Autodesk Inventor part; units mm, degrees
ref_plane "Work Plane1" through (15.7004, 0, 0) normal (0, -1, 0) x (1, 0, 0)
ref_plane "YZ Plane" through (0, 0, 0) normal (1, 0, 0) x (0, 1, 0)
ref_plane "XZ Plane" through (0, 0, 0) normal (0, 1, 0) x (-1, 0, 0)
sketch "Sketch1" plane through (0, 0, 0) normal (0, 0, 1) x (1, 0, 0)
  arc A0 (-20.5392, 17.1146) -> (-21.125, 15.7004) centre (-19.125, 15.7004) ccw
  line L0 (-21.125, -15.7004) -> (-21.125, 15.7004)
  arc A1 (-21.125, -15.7004) -> (-20.5392, -17.1146) centre (-19.125, -15.7004) ccw
  line L1 (-20.5392, -17.1146) -> (-17.1146, -20.5392)
  arc A2 (-17.1146, -20.5392) -> (-15.7004, -21.125) centre (-15.7004, -19.125) ccw
  line L2 (15.7004, -21.125) -> (-15.7004, -21.125)
  arc A3 (15.7004, -21.125) -> (17.1146, -20.5392) centre (15.7004, -19.125) ccw
  line L3 (20.5392, -17.1146) -> (17.1146, -20.5392)
  arc A4 (20.5392, -17.1146) -> (21.125, -15.7004) centre (19.125, -15.7004) ccw
  line L4 (21.125, 15.7004) -> (21.125, -15.7004)
  arc A5 (21.125, 15.7004) -> (20.5392, 17.1146) centre (19.125, 15.7004) ccw
  line L5 (20.5392, 17.1146) -> (17.1146, 20.5392)
  arc A6 (17.1146, 20.5392) -> (15.7004, 21.125) centre (15.7004, 19.125) ccw
  line L6 (-15.7004, 21.125) -> (15.7004, 21.125)
  arc A7 (-15.7004, 21.125) -> (-17.1146, 20.5392) centre (-15.7004, 19.125) ccw
  line L7 (-20.5392, 17.1146) -> (-17.1146, 20.5392)
  circle A8 centre (0, 0) radius 16
  circle A9 centre (-15.875, -15.875) radius 1.625
  circle A10 centre (15.875, 15.875) radius 1.625
  circle A11 centre (-15.875, 15.875) radius 1.625
  circle A12 centre (15.875, -15.875) radius 1.625
  circle A13 centre (0, 0) radius 11
  point P0 (0, 0)
extrude "Extrusion1" add sketch "Sketch1" along normal blind 5 contours L7 A7 L6 A6 L5 A5 L4 A4 L3 A3 L2 A2 L1 A1 L0 A0 | A8
sketch "Sketch2" plane through (-21.125, -15.7004, 0) normal (-1, 0, 0) x (0, 0, 1)
  line L0 (0, -5.4246) -> (5, -5.4246)
  line L1 (5, -5.4246) -> (-28, -5.4246)
  line L2 (-28, -5.4246) -> (-28, 36.8254)
  line L3 (-28, 36.8254) -> (5, 36.8254)
  line L4 (5, 36.8254) -> (5, -5.4246)
  point P0 (0, 15.7004)
  dimension "d6" = 33
extrude "Extrusion2" add sketch "Sketch2" along normal blind 5
sketch "Sketch3" plane through (0, 0, 5) normal (0, 0, 1) x (1, 0, 0)
  line L0 (-21.125, -15.7004) -> (-21.125, -21.125)
  arc A0 (-21.125, -15.7004) -> (-20.5392, -17.1146) centre (-19.125, -15.7004) ccw
  arc A1 (-17.1146, -20.5392) -> (-15.7004, -21.125) centre (-15.7004, -19.125) ccw
  line L1 (-20.5392, -17.1146) -> (-17.1146, -20.5392)
  line L2 (-21.125, -21.125) -> (-15.7004, -21.125)
  line L3 (-21.125, 21.125) -> (-21.125, 15.7004)
  arc A2 (-15.7004, 21.125) -> (-17.1146, 20.5392) centre (-15.7004, 19.125) ccw
  line L4 (-21.125, 21.125) -> (-15.7004, 21.125)
  line L5 (-17.1146, 20.5392) -> (-20.5392, 17.1146)
  arc A3 (-20.5392, 17.1146) -> (-21.125, 15.7004) centre (-19.125, 15.7004) ccw
  point P0 (0, 0)
extrude "Extrusion3" add sketch "Sketch3" against normal blind 5
sketch "Sketch4" plane through (-26.125, -15.7004, 0) normal (-1, 0, 0) x (0, 0, 1)
  line L0 (0, -5.4246) -> (-28, -5.4246)
  line L1 (5, 36.8254) -> (-28, 36.8254)
  line L2 (-28, -5.4246) -> (-23, -5.4246)
  line L3 (-23, -5.4246) -> (-23, 36.8254)
  line L4 (-23, 36.8254) -> (-28, 36.8254)
  line L5 (-28, 36.8254) -> (-28, -5.4246)
  point P0 (0, 15.7004)
  dimension "d7" = 5
extrude "Extrusion4" add sketch "Sketch4" along normal blind 15
sketch "Sketch5" plane through (-26.125, -21.125, -23) normal (0, 0, 1) x (1, 0, 0)
  circle A0 centre (-5, 32.25) radius 2.25
  circle A1 centre (-5, 10) radius 2.25
  line L0 (0, 42.25) -> (-15, 42.25)
  line L1 (-15, 0) -> (-15, 42.25)
  line L2 (0, 0) -> (-15, 0)
  point P0 (26.125, 21.125)
  dimension "d10" = 10
  dimension "d11" = 10
  dimension "d12" = 10
  dimension "d13" = 10
  dimension "d14" = 4.5
  dimension "d15" = 4.5
extrude "Extrusion5" cut sketch "Sketch5" along normal through all both and the other way through all
ref_plane "Work Plane1" through (15.7004, 0, 0) normal (0, -1, 0) x (1, 0, 0)
sketch "Sketch6" plane through (15.7004, 0, 0) normal (0, -1, 0) x (1, 0, 0)
  line L0 (-41.8254, -23) -> (-56.8254, -23)
  line L1 (0, 5) -> (-41.8254, 5)
  line L2 (-56.8254, -23) -> (-41.8254, 5)
  line L3 (-41.8254, 5) -> (-41.8254, -23)
  line L4 (-41.8254, -23) -> (-56.8254, -23)
  point P0 (-15.7004, 0)
extrude "Extrusion6" add sketch "Sketch6" along normal mid plane 10
equation "\"d15\" = d14"
properties part number "StepperZHolder"
Can you work these out from the model? Positions are in its coordinate system, mm. A direction names the side the tool comes from. Coordinates: 2 decimals unless noted, no trailing zeros. Loops run counter-clockwise (first coordinate to the right, second up) from the corner with the lowest first, then second, coordinate; pieces in that order, holes last. Notation, with made-up numbers: M -22,-27 L -12,-27 A23 ccw -12,-11 Z; hole C 71,8 d9. An arc over 180 degrees is marked long. Return JSON: item names as keys, results as strings. Group by question number.
Item 1: Imagine slicing it at B-B (x = 0). Please give me the cut outline in (y, z) (3 decimals), and give its area (3 significant figures).
Item 2: Thinking about a two-plate mould opening in X: for faces 4 (the flat face through (18.851, 18.803, 2.465)), 5 (the cylindrical face through (16.62, -14.43, 2.46)), 6 (the flat face through (-30, -5, -15)), which applies, released by +X, released by -X, zero draft, split by the parting line, or undercut?
Item 3: Imagine slicing it at C-C (x = -30). Please give me the cut outline in (y, z) (3 decimals).
Item 4: If I drill on L1, parallel to X at y = -17, z = 3 (3 decimals); L2, parallel to X at y = -17.5, z = -6.5 (3 decimals); L3, parallel to Z at x = -18, y = 18, over which ranges is the centre line in solid material (lowest first)? Write a range as from..to.
Item 5: Imagine slicing it at D-D (z = -21.5). Please give me the cut outline in (x, y) (3 decimals), and give its area (3 significant figures).
Item 6: Imagine slicing it at A-A (y = 0). Please give me the cut outline in (x, z) (3 decimals).
Item 7: On a 3-axis mill with a long thin cutter (end or side, diameter ignored), from which of +Z, -Z, +X, -X, +Y, -Y can I reach the whole of each face in a straight line? I mean faces 1 (the flat face through (-34, 13, -23)), 2 (the flat face through (-10, 10, 0)), 3 (the flat face through (-34, -13, -23)). Say none if no direction works.
Item 8: I'm going to push flat-ended pins straight in: pin 1 Ø4.5 at (x, y) = (-32.5, -12.5) entering from +Z; pin 2 Ø5 at (y, z) = (10.5, -10.5) entering from -X (3 decimals); pin 3 Ø8 at (y, z) = (16, -12.5) entering from +X (3 decimals); pin 4 Ø2.5 at (x, y) = (15.875, -15.875) entering from -Z. Where does each tip first touch, or does it pass through?
Verdict:
{
 "1": {"outline": "M -21.125,0 L -11,0 L -11,5 L -21.125,5 Z; M 11,0 L 21.125,0 L 21.125,5 L 11,5 Z", "area": "101 mm^2"},
 "2": {"face 4": "released by +X", "face 5": "undercut", "face 6": "zero draft"},
 "3": {"outline": "M -21.125,-28 L -13.074,-28 L -13.074,-23 L -21.125,-23 Z; M -9.176,-28 L 9.176,-28 L 9.176,-23 L 5,-23 L 5,-2.233 L -5,-2.233 L -5,-23 L -9.176,-23 Z; M 13.074,-28 L 21.125,-28 L 21.125,-23 L 13.074,-23 Z"},
 "4": {"L1": "x = -26.125..-17.048, -14.702..14.702, 17.048..20.645", "L2": "x = -26.125..-21.125", "L3": "z = 0..5"},
 "5": {"outline": "M -40.321,-5 L -26.125,-5 L -26.125,-21.125 L -21.125,-21.125 L -21.125,21.125 L -26.125,21.125 L -26.125,5 L -40.321,5 Z", "area": "353 mm^2"},
 "6": {"outline": "M -41.125,-28 L -21.125,-28 L -21.125,0 L -11,0 L -11,5 L -26.125,5 L -41.125,-23 Z; M 11,0 L 21.125,0 L 21.125,5 L 11,5 Z"},
 "7": {"face 1": "+Z, -X, +Y", "face 2": "-Z, +X, +Y, -Y", "face 3": "+Z, -X, -Y"},
 "8": {"pin 1": "stops at z = -23", "pin 2": "stops at x = -26.125", "pin 3": "stops at x = -21.125", "pin 4": "passes through"}
}
